Study the drawing (mm; zero at the part's minimum x, y, z) and answer. Round coordinates to 2 decimals unless told otherwise and drop trailing zeros. Write each loop counter-clockwise with the first axis right and the second up, starting at its lowest first coordinate (ties: lowest second). Pieces come first, ordered by that corner, then holes. Notation, with made-up numbers: (78, 87.25) - (115, 87.25) arc R25 cw to (115, 119.25) - close; hole circle Ø4 at (82, 74). An arc over 180 degrees is marked (long way). Use one line per item in the form item = value. Start each with the question number.
1) Consider line 1 along X through (y, z) = (67.5, 1) (1 decimal); line 2 along Y through (x, z) = (13.5, 1); line 3 along Z through (x, y) = (4.5, 30.5) (1 decimal). Determine where each line is inside the solid, lowest interval first. Write a range as from..to.
2) The part is cut by section A-A, the plane x = 3.81. Give the vertices of the cut face in (y, z), plus the area to 3 significant figures.
3) Each of these flat-tipped pins is pushed along its axis until it touches: pin 1 (2.5 mm diameter, centred on x = 3.99, y = 68.07, fed in from +Z); pin 2 (5 mm diameter, centred on x = 26.5, z = 5, fed in from -Y). Where does it stop, or does it pass through?
4) The part is cut by section B-B, the plane y = 24. Give the vertices of the cut face in (x, z).
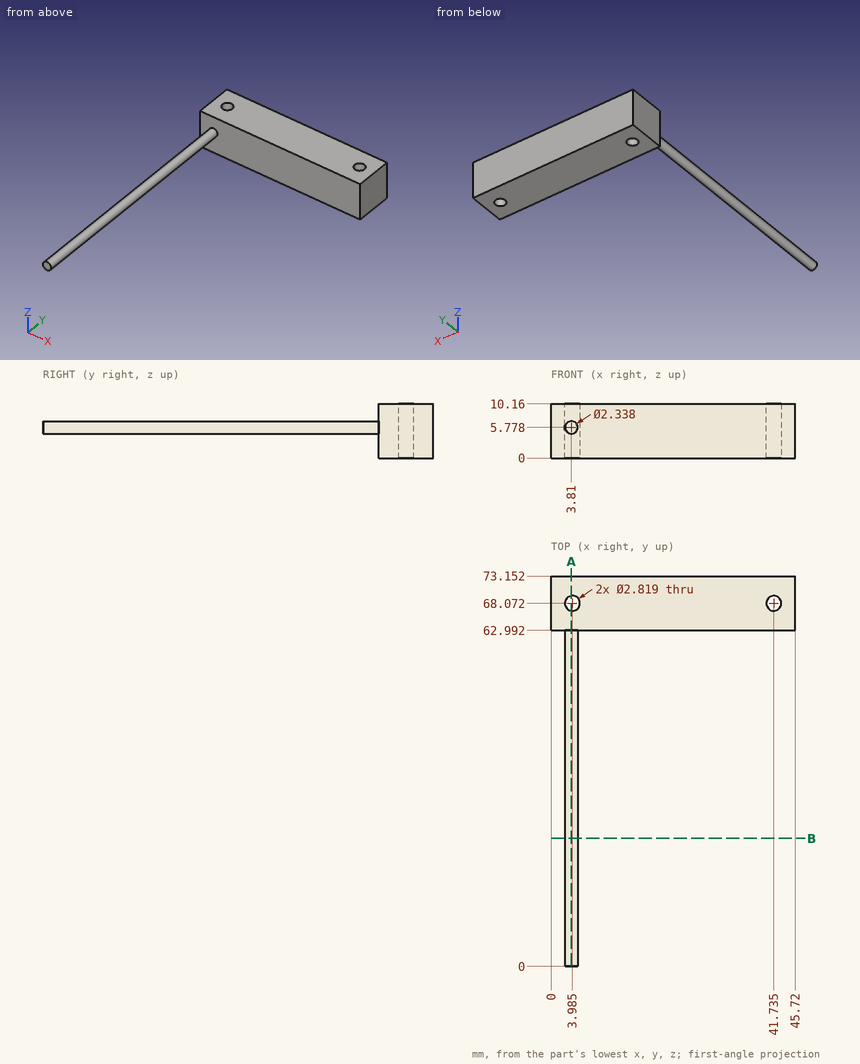
Geometry results:
q1.line_1 = 0..2.7, 5.3..40.4, 43..45.7
q1.line_2 = 62.99..73.15
q1.line_3 = 4.8..6.7
q2.outline = (0, 4.61) - (62.99, 4.61) - (62.99, 0) - (66.67, 0) - (66.67, 10.16) - (62.99, 10.16) - (62.99, 6.95) - (0, 6.95) - close; (69.47, 0) - (73.15, 0) - (73.15, 10.16) - (69.47, 10.16) - close
q2.area = 222 mm2
q3.pin_1 = through
q3.pin_2 = 62.99
q4.outline = circle Ø2.34 at (3.81, 5.78)
